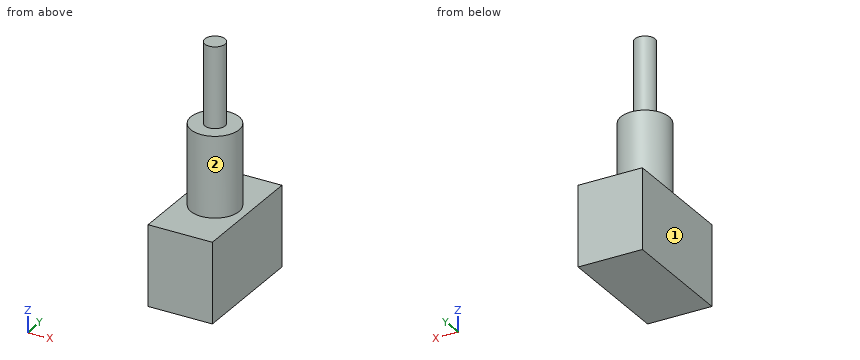
from build123d import *

# Parameters (mm, degrees)
F0_W     = 8
F0_H     = 15
F1_DEPTH = 10
F2_R     = 3
F3_DEPTH = 10
F4_R     = 1.25
F5_DEPTH = 10


with BuildPart() as f1:
    # F0 (on Top) → F1 (new body)
    with BuildSketch(Plane.XY):
        Rectangle(F0_W, F0_H)
    extrude(amount=F1_DEPTH)

    # F2 (on face) → F3 (join)
    with BuildSketch(Plane.XY.offset(10)):
        Circle(F2_R)
    extrude(amount=F3_DEPTH)

    # F4 (on face) → F5 (join)
    with BuildSketch(Plane.XY.offset(20)):
        Circle(F4_R)
    extrude(amount=F5_DEPTH)


solid = f1.part
Can you work these out from the model? Positions are in its coordinate system, mm. Face numbers are marked on the shaded views. A direction names the side the tool comes from. Coordinates: 2 decimals unless noted, no trailing zeros. Write each loop counter-clockwise with the first axis right and the second up, starting at its lowest first coordinate (ties: lowest second). Pieces come first, ordered by that corner, then holes. Notation, with made-up numbers: (66, 89.25) - (112, 89.25) arc R18 ccw to (112, 104.25) - close; hole circle Ø4 at (-17.75, 12.25). An arc over 180 degrees is marked (long way). Return JSON: item names as keys, results as strings. Group by question number.
Item 1: If we section it at B-B (y = 0): Write out the boundary of the cut face in (x, z), then the cut area to 3 significant figures.
Item 2: If we section it at D-D (z = 22.75): Write out the boundary of the cut face in (x, y), then the cut area to 3 significant figures.
Item 3: Which directions (+Z, -Z, +X, -X, +Y, -Y) give clear straight access to the entire face, cutting with the end or side of a thin tool? Please do the marked faces 1 and 2.
Item 4: If we section it at C-C (z = 19.5): Write out the boundary of the cut face in (x, y).
Item 5: If we section it at A-A (x = 0): Write out the boundary of the cut face in (y, z).
Item 6: Please list where these lines run through material, in increasing order: probe 1 along Z at (x, y) = (3.25, -0.25); probe 2 along Z at (x, y) = (-2.5, 1); probe 3 along X at (y, z) = (2.75, 17).
Item 7: I'm going to push flat-ended pins straight in: pin 1 Ø4 at (x, z) = (1.5, 18) entering from +Y; pin 2 Ø3 at (x, y) = (3, 3) entering from -Z. Where does each tip first touch, or does it pass through?
Return value:
{
 "1": {"outline": "(-4, 0) - (4, 0) - (4, 10) - (3, 10) - (3, 20) - (1.25, 20) - (1.25, 30) - (-1.25, 30) - (-1.25, 20) - (-3, 20) - (-3, 10) - (-4, 10) - close", "area": "165 mm^2"},
 "2": {"outline": "circle Ø2.5 at (0, 0)", "area": "4.91 mm^2"},
 "3": {"face 1": "+Z, -Z, -X, +Y, -Y", "face 2": "+Z"},
 "4": {"outline": "circle Ø6 at (0, 0)"},
 "5": {"outline": "(-7.5, 0) - (7.5, 0) - (7.5, 10) - (3, 10) - (3, 20) - (1.25, 20) - (1.25, 30) - (-1.25, 30) - (-1.25, 20) - (-3, 20) - (-3, 10) - (-7.5, 10) - close"},
 "6": {"probe 1": "z = 0 to 10", "probe 2": "z = 0 to 20", "probe 3": "x = -1.2 to 1.2"},
 "7": {"pin 1": "stops at y = 3", "pin 2": "stops at z = 0"}
}
